CAD build for the part. Positions are in the model's coordinates, mm. A direction names the side the tool comes from. Round coordinates to 2 decimals unless told otherwise and drop trailing zeros. Write each loop counter-clockwise with the first axis right and the second up, starting at its lowest first coordinate (ties: lowest second). Pieces come first, ordered by that corner, then holes. Notation, with made-up numbers: (27.25, 47.25) -> (83.25, 47.25) arc R24 cw to (83.25, 78.25) -> close; hole circle Ø2 at (-3, 8). An arc over 180 degrees is marked (long way). Put each result on its own line as item: value. Start each with the question number.
1. Saw through at C-C on x = 76.75. List the corners of the cut face in (y, z).
2. Saw through at A-A on z = 74.5. List the corners of the cut face in (x, y), and give its area (3 significant figures).
3. Saw through at D-D on x = 68. List the corners of the cut face in (y, z).
4. 3-axis set-ups, long thin cutter, end or side, ignore diameter. For faces 4 (the flat face through (61, 114.591, 74)), 5 (the cylindrical face through (59.603, 113.824, 74.896)), 6 (the flat face through (61, 113.991, 74)): which of +Z, -Z, +X, -X, +Y, -Y reach the whole face in a straight line?
5. Pull direction X, two halves, no side cores. Call faces 1 (the flat face through (59, 113.991, 74)), 2 (the cylindrical face through (59.127, 114.287, 75.262)), 3 (the cylindrical face through (61.67, 113.73, 74.34)): pulls with the +X half, pulls with the -X half, needs draft (parallel to the pull), parting line crosses it, or undercut.
6. Flat gauge pin, fed straight in: P1, Ø0.6, axis at x = 60.5, z = 74.5, coming from the -Y side. Where does the tip first touch, or does it go through?
7. Saw through at B-B on y = 114.4. List the corners of the cut face in (x, z), and give its area (3 significant figures).
8. Drill centre lines: line 1 (Y direction, x = 62.5, z = 74.75); line 2 (Y direction, x = 81.5, z = 74.5); line 3 (X direction, y = 113.7, z = 74). Where is each one in solid material? Low to high. Write a range as from..to.
from build123d import *

# Parameters (mm, degrees)
BOSS_EXTRUDE2_DEPTH = 0.18
SKETCH4_R           = 1
CUT_EXTRUDE1_DEPTH  = 1.18
SKETCH7_R           = 2
BOSS_EXTRUDE3_DEPTH = 0.6
SKETCH8_R           = 1.4
SKETCH8_R_2         = 1
BOSS_EXTRUDE4_DEPTH = 0.93


with BuildPart() as part:
    # Sketch2 → Boss-Extrude2 (new body)
    with BuildSketch(Plane.XZ.offset(-113.480952772)):
        with BuildLine():
            Line((60.372883835, 72.194540047), (70.125446667, 70.394451024))
            ThreePointArc((70.125446667, 70.394451024), (70.859385482, 70.238798062), (71.58406324, 70.044540047))
            Line((71.58406324, 70.044540047), (79.733100179, 67.627269484))
            ThreePointArc((79.733100179, 67.627269484), (81.847875106, 67.781237193), (83.333100179, 69.294540047))
            ThreePointArc((83.333100179, 69.294540047), (84.080389833, 71.617479067), (84.333100179, 74.044540047))
            ThreePointArc((84.333100179, 74.044540047), (84.080389833, 76.471601027), (83.333100179, 78.794540047))
            ThreePointArc((83.333100179, 78.794540047), (81.847875106, 80.307842901), (79.733100179, 80.46181061))
            Line((79.733100179, 80.46181061), (71.58406324, 78.044540047))
            ThreePointArc((71.58406324, 78.044540047), (70.859385482, 77.850282031), (70.125446667, 77.69462907))
            Line((70.125446667, 77.69462907), (60.372883835, 75.894540047))
            ThreePointArc((60.372883835, 75.894540047), (58.833100179, 74.044540047), (60.372883835, 72.194540047))
        make_face()
    extrude(amount=-BOSS_EXTRUDE2_DEPTH)

    # Sketch4 → Cut-Extrude1 (cut, through all)
    with BuildSketch(Plane.XZ.offset(-113.480952772)):
        with Locations((60.714349432, 74.044540047)):
            Circle(SKETCH4_R)
    extrude(amount=-CUT_EXTRUDE1_DEPTH, mode=Mode.SUBTRACT)



with BuildPart() as body_2:
    # Sketch7 → Boss-Extrude3 (new body)
    with BuildSketch(Plane(origin=(0, 113.990952772, 0), x_dir=(1, 0, 0), z_dir=(0, 1, 0))):
        with Locations((60.714349432, -74.044540047)):
            Circle(SKETCH7_R)
    extrude(amount=BOSS_EXTRUDE3_DEPTH)


with BuildPart() as part_1:
    add(part.part)

    add(body_2.part)  # Boss-Extrude4 merges body 2
    # Sketch8 → Boss-Extrude4 (add)
    with BuildSketch(Plane(origin=(0, 113.660952772, 0), x_dir=(1, 0, 0), z_dir=(0, 1, 0))):
        with Locations((60.714349432, -74.044540047)):
            Circle(SKETCH8_R)
        with Locations((60.714349432, -74.044540047)):
            Circle(SKETCH8_R_2, mode=Mode.SUBTRACT)
    extrude(amount=BOSS_EXTRUDE4_DEPTH)


solid = part_1.part
Return value:
1. outline: (113.48, 68.51) -> (113.66, 68.51) -> (113.66, 79.58) -> (113.48, 79.58) -> close
2. outline: (58.77, 113.99) -> (59.39, 113.99) -> (59.39, 113.66) -> (58.89, 113.66) -> (58.89, 113.48) -> (59.82, 113.48) -> (59.82, 113.99) -> (61.6, 113.99) -> (61.6, 113.48) -> (84.32, 113.48) -> (84.32, 113.66) -> (62.04, 113.66) -> (62.04, 113.99) -> (62.66, 113.99) -> (62.66, 114.59) -> (58.77, 114.59) -> close
2. area: 6.88 mm^2
3. outline: (113.48, 70.79) -> (113.66, 70.79) -> (113.66, 77.3) -> (113.48, 77.3) -> close
4. face 4: +Z, -Z, +X, -X, +Y
4. face 5: none
4. face 6: -Y
5. face 1: needs draft
5. face 2: parting line crosses it
5. face 3: undercut
6. P1: stops at y = 113.99
7. outline: circle Ø4 at (60.71, 74.04)
7. area: 12.6 mm^2
8. line 1: y = 113.48..113.66, 113.99..114.59
8. line 2: y = 113.48..113.66
8. line 3: x = 59.32..59.72, 61.71..62.11
